```python
from build123d import *

# Parameters (mm, degrees)
SKETCH1_W           = 350
SKETCH1_H           = 350
BOSS_EXTRUDE1_DEPTH = 10
SKETCH3_W           = 350
SKETCH3_H           = 76
CUT_EXTRUDE1_DEPTH  = 10
SKETCH4_W           = 25
SKETCH4_H           = 55
CUT_EXTRUDE2_DEPTH  = 10


with BuildPart() as part:
    # Sketch1 → Boss-Extrude1 (new body)
    with BuildSketch(Plane(origin=(0, 0, 0), x_dir=(1, 0, 0), z_dir=(0, 1, 0))):
        Rectangle(SKETCH1_W, SKETCH1_H)
    extrude(amount=BOSS_EXTRUDE1_DEPTH)

    # Sketch3 → Cut-Extrude1 (cut)
    with BuildSketch(Plane(origin=(0, 10, 0), x_dir=(1, 0, 0), z_dir=(0, 1, 0))):
        with Locations((0, -137)):
            Rectangle(SKETCH3_W, SKETCH3_H)
    extrude(amount=-CUT_EXTRUDE1_DEPTH, mode=Mode.SUBTRACT)

    # Sketch4 → Cut-Extrude2 (cut)
    with BuildSketch(Plane(origin=(0, 10, 0), x_dir=(1, 0, 0), z_dir=(0, 1, 0))):
        with Locations((0, 8.5)):
            Rectangle(SKETCH4_W, SKETCH4_H)
    extrude(amount=-CUT_EXTRUDE2_DEPTH, mode=Mode.SUBTRACT)


solid = part.part
```
CAD build for the part. Positions are in the model's coordinates, mm. A direction names the side the tool comes from. Coordinates: 2 decimals unless noted, no trailing zeros. Loops run counter-clockwise (first coordinate to the right, second up) from the corner with the lowest first, then second, coordinate; pieces in that order, holes last. Notation, with made-up numbers: (-26.75, -19.75) - (0.25, -19.75) arc R11 cw to (0.25, -15.75) - close; hole circle Ø2 at (87, 62.5). An arc over 180 degrees is marked (long way). Return JSON: item names as keys, results as strings.
1. Mould opens along Z. For faces 1 (the flat face through (-2, 5, -175)), 2 (the flat face through (12.5, 5, -8)), 3 (the flat face through (-2, 0, -40)), 4 (the flat face through (0, 5, -36)) say: released by +Z, released by -Z, zero draft, split by the parting line, or undercut.
Result:
{"face 1": "released by -Z", "face 2": "undercut", "face 3": "zero draft", "face 4": "undercut"}
2. Probe L1, parallel to X at y = 0.5, z = -7.5; L2, parallel to Z at x = 10, y = 4. List the from-to ranges inside material, lowest first. Write a range as from..to.
Result:
{"L1": "x = -175..-12.5, 12.5..175", "L2": "z = -175..-36, 19..99"}
3. Band-saw the part on B-B (z = -29). Give the cut face in (x, y).
Result:
{"outline": "(-175, 0) - (-12.5, 0) - (-12.5, 10) - (-175, 10) - close; (12.5, 0) - (175, 0) - (175, 10) - (12.5, 10) - close"}
4. Band-saw the part on A-A (x = 2). Give the cut face in (y, z), and give its area (3 significant figures).
Result:
{"outline": "(0, -175) - (10, -175) - (10, -36) - (0, -36) - close; (0, 19) - (10, 19) - (10, 99) - (0, 99) - close", "area": "2,190 mm2"}
5. 3-axis set-ups, long thin cutter, end or side, ignore diameter. For faces 5 (the flat face through (-12.5, 5, -8)), 6 (the flat face through (-2, 10, -40)): which of +Z, -Z, +X, -X, +Y, -Y reach the whole face in a straight line?
Result:
{"face 5": "+Y, -Y", "face 6": "+Z, -Z, +X, -X, +Y"}
